Part model, mm, in its own coordinate system. Coordinates: 2 decimals unless noted, no trailing zeros. Write each loop counter-clockwise with the first axis right and the second up, starting at its lowest first coordinate (ties: lowest second). Pieces come first, ordered by that corner, then holes. Notation, with made-up numbers: M 35,-13 L 65,-13 A30 cw 65,20 Z; hole C 12,74 d10. An arc over 180 degrees is marked long. Use a Markdown table: item, result. Add a question column.
Q1. Slice it at C-C on z = 14. Write the cut outline in (x, y), then the cut area to 3 significant figures.
Q2. Slice it at A-A on z = 0. Write the cut outline in (x, y) (3 decimals), then the cut area to 3 significant figures.
Q3. Slice it at D-D on z = 43. Write the cut outline in (x, y), then the cut area to 3 significant figures.
Q4. Wall check: L1, parallel to Z at x = -23.5, y = 1.5; L2, parallel to Z at x = 23, y = 2.5; L3, parallel to Z at x = 1.5, y = 1. Give the ranges that are in metal, low to high. Write a range as from..to.
Q5. Slice it at B-B on y = 2. Count the separate pieces of the cut face and the enclosed holes in it, then the cut area to 3 significant figures.
Q6. Pin check, flat tips, straight feed: pin 1 Ø4 at (x, z) = (-37.5, 37.5) entering from -Y; pin 2 Ø1 at (y, z) = (3, -18.5) entering from +X; pin 3 Ø2 at (y, z) = (4.5, 22.5) entering from -X; pin 4 Ø2 at (x, y) = (-14.5, 3) entering from +Z. Stop position of each tip, or through.
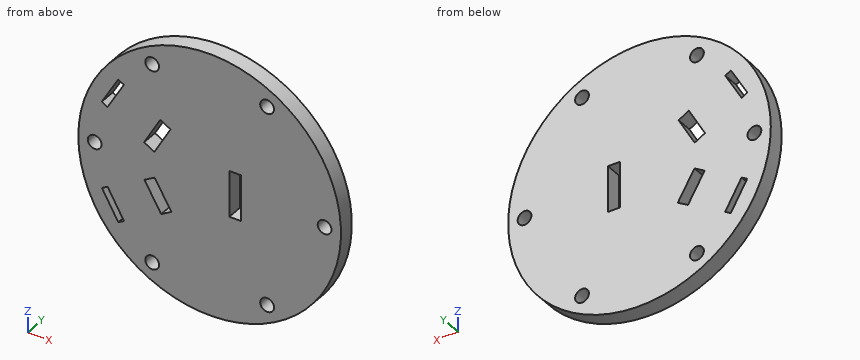
Autodesk Inventor part; units mm, degrees
ref_plane "YZ Plane" through (0, 0, 0) normal (1, 0, 0) x (0, 1, 0)
ref_plane "XZ Plane" through (0, 0, 0) normal (0, 1, 0) x (-1, 0, 0)
ref_plane "XY Plane" through (0, 0, 0) normal (0, 0, 1) x (1, 0, 0)
sketch "Sketch4" plane through (0, 0, 0) normal (0, 1, 0) x (-1, 0, 0)
  circle A0 centre (0, 0) radius 50.8
  dimension "d2" = 101.6
extrude "Extrusion3" add sketch "Sketch4" along normal blind 6.35
sketch "Sketch10" plane through (0, 6.35, 0) normal (0, 1, 0) x (1, 0, 0)
  circle A0 centre (-44.462, 0) radius 2.667
  circle A1 centre (-22.231, -38.5052) radius 2.667
  circle A2 centre (22.231, -38.5052) radius 2.667
  circle A3 centre (44.462, 0) radius 2.667
  circle A4 centre (22.231, 38.5052) radius 2.667
  circle A5 centre (-22.231, 38.5052) radius 2.667
  point P0 (0, 0)
  dimension "d48" = 5.334
  dimension "d51" = 360
extrude "Extrusion6" cut sketch "Sketch10" against normal blind 6.35
sketch "Sketch13" plane through (0, 6.35, 0) normal (0, 1, 0) x (1, 0, 0)
  line L0 (-25.3494, -7.0256) -> (-21.3685, -4.7771)
  line L1 (-21.3685, -4.7771) -> (-15.1225, -15.8349)
  line L2 (-15.1225, -15.8349) -> (-19.1033, -18.0835)
  line L3 (-19.1033, -18.0835) -> (-25.3494, -7.0256)
  line L4 (-25.3494, -7.0256) -> (-21.3685, -4.7771)
  line L5 (-21.3685, -4.7771) -> (-15.1225, -15.8349)
  line L6 (-15.1225, -15.8349) -> (-19.1033, -18.0835)
  line L7 (-19.1033, -18.0835) -> (-25.3494, -7.0256)
  line L8 (-25.3494, -7.0256) -> (-21.3685, -4.7771)
  line L9 (-21.3685, -4.7771) -> (-15.1225, -15.8349)
  line L10 (-15.1225, -15.8349) -> (-19.1033, -18.0835)
  line L11 (-19.1033, -18.0835) -> (-25.3494, -7.0256)
  line L12 (-25.3494, -7.0256) -> (-21.3685, -4.7771)
  line L13 (-21.3685, -4.7771) -> (-15.1225, -15.8349)
  line L14 (-15.1225, -15.8349) -> (-19.1033, -18.0835)
  line L15 (-19.1033, -18.0835) -> (-25.3494, -7.0256)
  line L16 (-25.3494, -7.0256) -> (-21.3685, -4.7771)
  line L17 (-21.3685, -4.7771) -> (-15.1225, -15.8349)
  line L18 (-15.1225, -15.8349) -> (-19.1033, -18.0835)
  line L19 (-19.1033, -18.0835) -> (-25.3494, -7.0256)
  line L20 (-25.3494, -7.0256) -> (-21.3685, -4.7771)
  line L21 (-21.3685, -4.7771) -> (-15.1225, -15.8349)
  line L22 (-15.1225, -15.8349) -> (-19.1033, -18.0835)
  line L23 (-19.1033, -18.0835) -> (-25.3494, -7.0256)
  line L24 (-18.7591, 18.4404) -> (-14.8213, 16.1172)
  line L25 (-14.8213, 16.1172) -> (-21.2747, 5.179)
  line L26 (-21.2747, 5.179) -> (-25.2124, 7.5022)
  line L27 (-25.2124, 7.5022) -> (-18.7591, 18.4404)
  line L28 (-18.7591, 18.4404) -> (-14.8213, 16.1172)
  line L29 (-14.8213, 16.1172) -> (-21.2747, 5.179)
  line L30 (-21.2747, 5.179) -> (-25.2124, 7.5022)
  line L31 (-25.2124, 7.5022) -> (-18.7591, 18.4404)
  line L32 (-18.7591, 18.4404) -> (-14.8213, 16.1172)
  line L33 (-14.8213, 16.1172) -> (-21.2747, 5.179)
  line L34 (-21.2747, 5.179) -> (-25.2124, 7.5022)
  line L35 (-25.2124, 7.5022) -> (-18.7591, 18.4404)
  line L36 (-18.7591, 18.4404) -> (-14.8213, 16.1172)
  line L37 (-14.8213, 16.1172) -> (-21.2747, 5.179)
  line L38 (-21.2747, 5.179) -> (-25.2124, 7.5022)
  line L39 (-25.2124, 7.5022) -> (-18.7591, 18.4404)
  line L40 (-18.7591, 18.4404) -> (-14.8213, 16.1172)
  line L41 (-14.8213, 16.1172) -> (-21.2747, 5.179)
  line L42 (-21.2747, 5.179) -> (-25.2124, 7.5022)
  line L43 (-25.2124, 7.5022) -> (-18.7591, 18.4404)
  line L44 (-18.7591, 18.4404) -> (-14.8213, 16.1172)
  line L45 (-14.8213, 16.1172) -> (-21.2747, 5.179)
  line L46 (-21.2747, 5.179) -> (-25.2124, 7.5022)
  line L47 (-25.2124, 7.5022) -> (-18.7591, 18.4404)
  line L48 (7.62, 9.652) -> (12.192, 9.652)
  line L49 (12.192, 9.652) -> (12.192, -8.128)
  line L50 (12.192, -8.128) -> (7.62, -8.128)
  line L51 (7.62, -8.128) -> (7.62, 9.652)
  line L52 (-41.7125, -16.7155) -> (-39.5128, -15.4455)
  line L53 (-39.5128, -15.4455) -> (-33.1628, -26.444)
  line L54 (-33.1628, -26.444) -> (-35.3625, -27.714)
  line L55 (-35.3625, -27.714) -> (-41.7125, -16.7155)
  line L56 (-35.3322, 27.7663) -> (-33.1325, 26.4963)
  line L57 (-33.1325, 26.4963) -> (-39.4825, 15.4978)
  line L58 (-39.4825, 15.4978) -> (-41.6822, 16.7678)
  line L59 (-41.6822, 16.7678) -> (-35.3322, 27.7663)
  point P0 (0, 0)
  dimension "d57" = 4.572
  dimension "d58" = 12.7
  dimension "d59" = 4.572
  dimension "d60" = 12.7
  dimension "d61" = 4.572
  dimension "d62" = 12.7
  dimension "d63" = 4.572
  dimension "d64" = 12.7
  dimension "d65" = 4.572
  dimension "d66" = 12.7
  dimension "d67" = 4.572
  dimension "d68" = 12.7
  dimension "d69" = 4.572
  dimension "d70" = 12.7
  dimension "d71" = 4.572
  dimension "d72" = 12.7
  dimension "d73" = 4.572
  dimension "d74" = 12.7
  dimension "d75" = 4.572
  dimension "d76" = 12.7
  dimension "d77" = 4.572
  dimension "d78" = 12.7
  dimension "d79" = 4.572
  dimension "d80" = 12.7
  dimension "d81" = 4.572
  dimension "d82" = 17.78
  dimension "d109" = 2.54
  dimension "d110" = 12.7
  dimension "d113" = 2.54
  dimension "d114" = 12.7
extrude "Extrusion8" cut sketch "Sketch13" against normal blind 6.35
properties part number "cap with wire cut"
Recorded:
| question | item | result |
|---|---|---|
| 1 | outline | M -48.83,0 L -21.41,0 L -21.41,6.35 L -48.83,6.35 Z; M -16.16,0 L 48.83,0 L 48.83,6.35 L -16.16,6.35 Z |
| 1 | area | 587 mm² |
| 2 | outline | M -50.8,0 L -47.129,0 L -47.129,6.35 L -50.8,6.35 Z; M -41.795,0 L 7.62,0 L 7.62,6.35 L -41.795,6.35 Z; M 12.192,0 L 41.795,0 L 41.795,6.35 L 12.192,6.35 Z; M 47.129,0 L 50.8,0 L 50.8,6.35 L 47.129,6.35 Z |
| 2 | area | 548 mm² |
| 3 | outline | M -27.05,0 L 27.05,0 L 27.05,6.35 L -27.05,6.35 Z |
| 3 | area | 344 mm² |
| 4 | L1 | -45.04..-40.85, -36.16..-10.4, -6.49..5.98, 10.3..36.16, 40.85..45.04 |
| 4 | L2 | -45.3..-41.06, -35.95..35.95, 41.06..45.3 |
| 4 | L3 | -50.78..50.78 |
| 5 | separate pieces | 1 |
| 5 | enclosed holes | 11 |
| 5 | area | 7,710 mm² |
| 6 | pin 1 | through |
| 6 | pin 2 | x = 47.5 |
| 6 | pin 3 | x = -46.03 |
| 6 | pin 4 | z = 48.97 |
